Geometry check sheet. Reference: the model listing, model coordinates, mm. Face numbers are marked on the shaded views. Round coordinates to 2 decimals unless told otherwise and drop trailing zeros. Write each loop counter-clockwise with the first axis right and the second up, starting at its lowest first coordinate (ties: lowest second). Pieces come first, ordered by that corner, then holes. Notation, with made-up numbers: (0, -6.5) - (6, -6.5) arc R26 cw to (6, 32.5) - close; hole circle Ø2 at (33, 33.25). An arc over 180 degrees is marked (long way). One line per question, with ' | ' between items. Start each with the question number.
from build123d import *

# Parameters (mm, degrees)
SKETCH157_R      = 3.5
EXTRUDE147_DEPTH = 10
EXTRUDE097_DEPTH = 26.64


with BuildPart() as extrude147:
    # Sketch157 → Extrude147 (new body)
    with BuildSketch(Plane(origin=(0, 280, 0), x_dir=(-1, 0, 0), z_dir=(0, 1, 0))):
        with Locations((-134, -3.64)):
            Circle(SKETCH157_R)
    extrude(amount=-EXTRUDE147_DEPTH)


with BuildPart() as battery_side:
    # Sketch106 → Extrude097 (new body)
    with BuildSketch(Plane(origin=(0, 0, -20.32), x_dir=(1, 0, 0), z_dir=(0, 0, -1))):
        Polygon((47, -278.5), (215, -278.5), (215, -276.5), (178.5, -276.5), (178.5, -277.5), (157.5, -277.5), (157.5, -276.5), (47, -276.5), align=None)
    extrude(amount=-EXTRUDE097_DEPTH)

    # Cut017: cut Extrude147
    add(extrude147.part, mode=Mode.SUBTRACT)


solid = battery_side.part
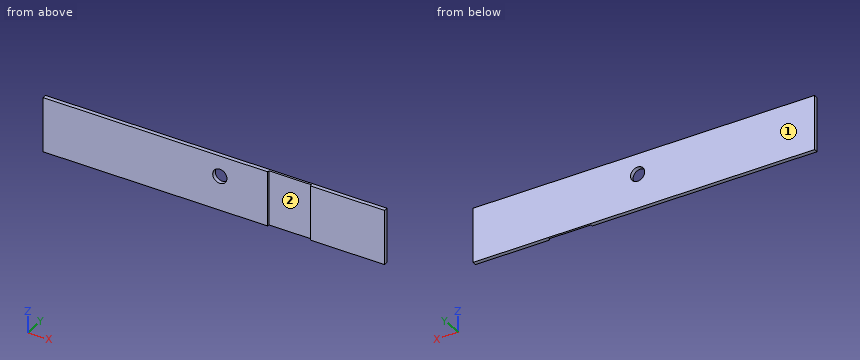
Q1. Section check C-C, the plane x = 134. Record the cut outline in (y, z).
Q2. Thickness scan on line 1 (Z direction, x = 134, y = 277.65); line 2 (X direction, y = 277.1, z = -10); line 3 (X direction, y = 276.9, z = -1). Record the ranges inside material, lowest first.
Q3. Section check B-B, the plane z = -17. Record the cut outline in (x, y), then the cut area to 3 significant figures.
Q4. Go/stop test with flat-tipped pins: P1, Ø10.5, axis at x = 169, z = -2.5, coming from the -Y side; P2, Ø6.5, axis at x = 134, z = -3.64, coming from the +Y side. Record where each tip stops, or that it passes through.
Q5. Section check A-A, the plane y = 277.05. Record the cut outline in (x, z).
Q6. Draft check along X on the marked faces 1 and 2. Enter one of: pulls with the +X half, pulls with the -X half, needs draft (parallel to the pull), parting line crosses it, or undercut.
Q7. Section check D-D, the plane z = -3.64. Record the cut outline in (x, y), then the cut area to 3 significant figures.
Result sheet:
1) outline: (276.5, -20.32) - (278.5, -20.32) - (278.5, -7.14) - (276.5, -7.14) - close; (276.5, -0.14) - (278.5, -0.14) - (278.5, 6.32) - (276.5, 6.32) - close
2) line 1: -20.32 to -7.14, -0.14 to 6.32 | line 2: 47 to 157.5, 178.5 to 215 | line 3: 47 to 131.7, 136.3 to 157.5, 178.5 to 215
3) outline: (47, 276.5) - (157.5, 276.5) - (157.5, 277.5) - (178.5, 277.5) - (178.5, 276.5) - (215, 276.5) - (215, 278.5) - (47, 278.5) - close | area: 315 mm²
4) P1: y = 277.5 | P2: through
5) outline: (47, -20.32) - (157.5, -20.32) - (157.5, 6.32) - (47, 6.32) - close; (178.5, -20.32) - (215, -20.32) - (215, 6.32) - (178.5, 6.32) - close; hole circle Ø7 at (134, -3.64)
6) face 1: needs draft | face 2: undercut
7) outline: (47, 276.5) - (130.5, 276.5) - (130.5, 278.5) - (47, 278.5) - close; (137.5, 276.5) - (157.5, 276.5) - (157.5, 277.5) - (178.5, 277.5) - (178.5, 276.5) - (215, 276.5) - (215, 278.5) - (137.5, 278.5) - close | area: 301 mm²
